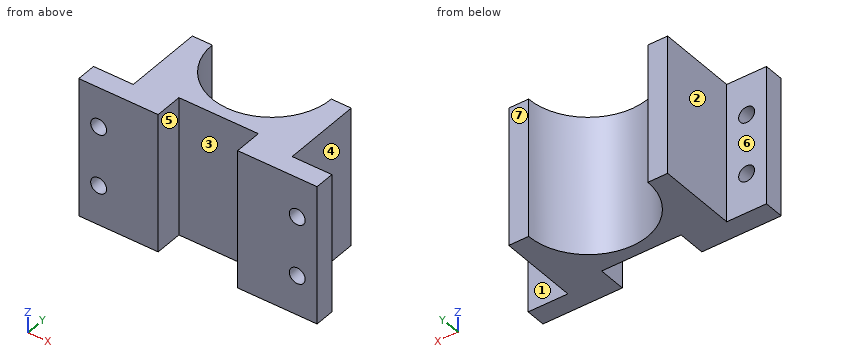
from build123d import *

# Parameters (mm, degrees)
IZIM1_W                     = 60
IZIM1_H                     = 25
Y_KSEKLIK_EKSTR_ZYON1_DEPTH = 35
IZIM2_W                     = 10
IZIM2_H                     = 20
IZIM2_W_2                   = 20
IZIM2_H_2                   = 7
KES_EKSTR_ZYON2_DEPTH       = 36
IZIM3_R                     = 2
KES_EKSTR_ZYON3_DEPTH       = 6


with BuildPart() as part:
    # Çizim1 → Yükseklik-Ekstrüzyon1 (new body)
    with BuildSketch(Plane.XY):
        with Locations((30, 12.5)):
            Rectangle(IZIM1_W, IZIM1_H)
    extrude(amount=Y_KSEKLIK_EKSTR_ZYON1_DEPTH)

    # Çizim2 → Kes-Ekstrüzyon2 (cut, through all)
    with BuildSketch(Plane.XY.offset(35)):
        with Locations((55, 15)):
            Rectangle(IZIM2_W, IZIM2_H)
        with BuildLine():
            Line((45, 25), (15, 25))
            ThreePointArc((15, 25), (30, 10), (45, 25))
        make_face()
        with Locations((5, 15)):
            Rectangle(IZIM2_W, IZIM2_H)
        with Locations((30, 3.5)):
            Rectangle(IZIM2_W_2, IZIM2_H_2)
    extrude(amount=-KES_EKSTR_ZYON2_DEPTH, mode=Mode.SUBTRACT)

    # Çizim3 → Kes-Ekstrüzyon3 (cut, through all)
    with BuildSketch(Plane(origin=(0, 5, 0), x_dir=(1, 0, 0), z_dir=(0, 1, 0))):
        with Locations((5, -25)):
            Circle(IZIM3_R)
        with Locations((5, -10)):
            Circle(IZIM3_R)
        with Locations((55, -10)):
            Circle(IZIM3_R)
        with Locations((55, -25)):
            Circle(IZIM3_R)
    extrude(amount=-KES_EKSTR_ZYON3_DEPTH, mode=Mode.SUBTRACT)


solid = part.part
For this review, take the finished solid that the model builds, in its own axes (mm). Face numbers are marked on the shaded views. A direction names the side the tool comes from. Give positions to 0.01 mm unless a question says otherwise; leave off trailing zeros. Loops run counter-clockwise (first coordinate to the right, second up) from the corner with the lowest first, then second, coordinate; pieces in that order, holes last. Notation, with made-up numbers: (53.25, 57.5) - (106.25, 57.5) arc R20 ccw to (106.25, 86.5) - close; hole circle Ø3 at (-9, 52). An arc over 180 degrees is marked (long way). Write each question's results on one line, items separated by ' | '.
(1) For the marked faces 5, 6 and 7, list the 3-axis set-ups (+Z, -Z, +X, -X, +Y, -Y) from which the entire face can be reached by the end or side of a thin tool; tool diameter is ignored.
Conclusion:
face 5: +Z, -Z, -Y | face 6: +Z, -Z, -X, +Y | face 7: +Z, -Z, +X, -X, +Y
(2) For line 1 along X through (y, z) = (2.15, 10); line 2 along Z through (x, y) = (55, 2.35); line 3 along Y through (x, z) = (52, 15), list the stretches that pass through material, from the lowest coordinate up.
Conclusion:
line 1: 0 to 3, 7 to 20, 40 to 53, 57 to 60 | line 2: 0 to 8, 12 to 23, 27 to 35 | line 3: 0 to 5
(3) Take a section at B-B (y = 16). Give the boundary of the cut face in (x, z).
Conclusion:
outline: (10, 0) - (18, 0) - (18, 35) - (10, 35) - close; (42, 0) - (50, 0) - (50, 35) - (42, 35) - close
(4) Take a section at D-D (z = 33). Give the boundary of the cut face in (x, y).
Conclusion:
outline: (0, 0) - (20, 0) - (20, 7) - (40, 7) - (40, 0) - (60, 0) - (60, 5) - (50, 5) - (50, 25) - (45, 25) arc R15 cw to (15, 25) - (10, 25) - (10, 5) - (0, 5) - close
(5) For pin 1 Ø5 at (y, z) = (21, 28.5) entering from -X; pin 2 Ø6 at (x, z) = (38.5, 8) entering from +Y; pin 3 Ø5 at (y, z) = (13.5, 11.5) entering from +X; pin 4 Ø3 at (x, z) = (5, 25) entering from -Y, all flat-tipped, find the tip position at first contact; note any pin that passes through.
Conclusion:
pin 1: x = 10 | pin 2: y = 15.37 | pin 3: x = 50 | pin 4: through
(6) Draft analysis for pull direction X (two halves, no side actions). For the marked faces 1, 2, 3 and 4, state which applies: +X half, -X half, draft (parallel to the pull), parting line (faces both ways), or undercut.
Conclusion:
face 1: draft | face 2: -X half | face 3: undercut | face 4: +X half
(7) Take a section at C-C (z = 25). Give the boundary of the cut face in (x, y).
Conclusion:
outline: (0, 0) - (3, 0) - (3, 5) - (0, 5) - close; (7, 0) - (20, 0) - (20, 7) - (40, 7) - (40, 0) - (53, 0) - (53, 5) - (50, 5) - (50, 25) - (45, 25) arc R15 cw to (15, 25) - (10, 25) - (10, 5) - (7, 5) - close; (57, 0) - (60, 0) - (60, 5) - (57, 5) - close
(8) Take a section at A-A (x = 5). Give the boundary of the cut face in (y, z), then the cut area to 3 significant figures.
Conclusion:
outline: (0, 0) - (5, 0) - (5, 8) - (0, 8) - close; (0, 12) - (5, 12) - (5, 23) - (0, 23) - close; (0, 27) - (5, 27) - (5, 35) - (0, 35) - close | area: 135 mm^2
